Build history of the part. All positions in model axes, mm. A direction names the side the tool comes from. Round coordinates to 2 decimals unless told otherwise and drop trailing zeros. Order: outer loops, then holes, each group sorted by start corner. A loop starts at its lowest first (then second) coordinate and runs counter-clockwise, first axis right, second up. Notation, with made-up numbers: (65, 75) -> (77, 75) arc R31 ccw to (77, 104) -> close; hole circle Ø4 at (32, 3). An arc over 180 degrees is marked (long way). Answer as a JSON object with one key per item and string values.
Autodesk Fusion 360 part; units mm, degrees
sketch "スケッチ1" plane through (0, 0, 0) normal (0, 0, 1) x (1, 0, 0)
  circle A0 centre (0, 0) radius 10
  line L0 (0, 10) -> (12, 10)
  line L1 (12, 10) -> (12, 22)
  line L2 (19, 22) -> (19, -16)
  line L3 (12, -20) -> (12, -10)
  line L4 (12, -10) -> (0, -10)
  line L5 (0, -7) -> (0, 7)
  line L6 (19, -7) -> (14, -7)
  line L7 (14, -7) -> (14, 7)
  line L8 (14, 7) -> (19, 7)
  line L9 (12, 22) -> (19, 22)
  line L10 (12, -20) -> (27, -20)
  line L11 (27, -20) -> (27, -13)
  line L12 (27, -13) -> (23, -13)
  line L13 (23, -13) -> (23, -16)
  line L14 (23, -16) -> (19, -16)
  point P0 (14, 0)
  dimension "d1" = 20
  dimension "d2" = 12
  dimension "d6" = 7
  dimension "d19" = 14
  dimension "d31" = 5
  dimension "d32" = 14
  dimension "d39" = 22
  dimension "d40" = 13
  dimension "d41" = 3
  dimension "d42" = 4
  dimension "d43" = 4
  dimension "d44" = 4
extrude "押し出し1" add sketch "スケッチ1" along normal blind 8 contours A0 | A0 L0 L1 L2 L3 L4 L6 L7 L8 L9 L10 L11 L12 L13 L14
sketch "スケッチ2" plane through (0, 0, 8) normal (0, 0, 1) x (-1, 0, 0)
  circle A0 centre (0, 0) radius 10
  line L0 (-12, 20) -> (-27, 20)
  line L1 (-27, 20) -> (-27, 13)
  line L2 (-27, 13) -> (-23, 13)
  line L3 (-23, 13) -> (-23, 16)
  line L4 (-23, 16) -> (-19, 16)
  line L5 (-19, 16) -> (-19, 7)
  line L6 (-19, -22) -> (-12, -22)
  line L7 (-12, -22) -> (-12, -10)
  line L8 (-12, -10) -> (0, -10)
  arc A1 (0, -10) -> (0, 10) centre (0, 0) ccw
  line L9 (0, 10) -> (-12, 10)
  line L10 (-12, 10) -> (-12, 20)
  line L11 (-19, 7) -> (-14, 7)
  line L12 (-14, 7) -> (-14, -7)
  line L13 (-14, -7) -> (-19, -7)
  line L14 (-19, -7) -> (-19, -22)
extrude "押し出し2" add sketch "スケッチ2" along normal blind 2.5 contours A0 A1
hole "穴1" at (0, 7, 0) at (0, -7, 0) direction (0, 0, 1) diameter 3.2 end through all
hole "穴3" at (0, 0, 0) direction (0, 0, 1) diameter 8 end through all
sketch "スケッチ3" plane through (0, -10, 0) normal (0, -1, 0) x (1, 0, 0)
  line L0 (0, 0) -> (12, 0)
  line L1 (12, 0) -> (12, 8)
  line L2 (12, 8) -> (0, 8)
  line L3 (0, 8) -> (0, 0)
  line L4 (10, 0) -> (4, 4)
  line L5 (4, 4) -> (-15, 4)
  line L6 (-15, 4) -> (-15, 0)
  line L7 (-15, 0) -> (10, 0)
  dimension "d20" = 10
  dimension "d21" = 15
  dimension "d22" = 6
  dimension "d23" = 4
extrude "押し出し3" cut sketch "スケッチ3" against normal through all contours L0 L3 L4 L5 L7 | L3 L5 L6 L7
sketch "スケッチ4" plane through (19, 0, 0) normal (1, 0, 0) x (0, 1, 0)
  line L0 (7, 0) -> (22, 0)
  line L1 (22, 8) -> (7, 8)
  line L2 (22, 4) -> (18, 4)
  line L3 (22, 0) -> (22, 8)
  line L4 (-16, 8) -> (-16, 0)
  line L5 (7, 8) -> (7, 0)
  line L6 (-16, 0) -> (-7, 0)
  line L7 (-7, 0) -> (-7, 8)
  line L8 (-7, 8) -> (-16, 8)
  dimension "d45" = 4
hole "穴2" at (19, 18, 4) direction (-1, 0, 0) diameter 3 depth 11 tip angle 118
thread "ねじ1"
fillet "フィレット1" radius 4 4 edges at (12, 10, 4) (12, -10, 4) (14, -7, 4) (14, 7, 4)
chamfer "面取り2" distance 1 angle 45 1 edges at (23, -13, 4)
1) Cut at D-D, the plane y = 4.5. Give the cut face in (x, z).
Checked values:
{"outline": "(-8.93, 4) -> (4, 4) -> (10, 0) -> (14.29, 0) -> (14.29, 8) -> (8.93, 8) -> (8.93, 10.5) -> (-8.93, 10.5) -> close"}
2) Which spindle directions (+Z, -Z, +X, -X, +Y, -Y) get a long thin tool onto all of the face, cutting with end or side? Do faces 1 (the face through (12, 20, 4)), 2 (the face through (15.203, 5.859, 4.056)), 3 (the face through (19, -11, 4)), 4 (the face through (-4.5, -0.1, 4)), 5 (the face through (5, -10, 5)). Say none if no direction does.
Checked values:
{"face 1": "+Z, -Z, -X, +Y", "face 2": "+Z, -Z, +X", "face 3": "+Z, -Z, +Y", "face 4": "-Z, -X, +Y, -Y", "face 5": "+Z, -Z, -X, -Y"}
3) Flat gauge pins, fed straight in: pin 1 Ø2 at (x, z) = (-0.5, 9.5) entering from +Y; pin 2 Ø1.5 at (x, y) = (14, -1.5) entering from +Z; pin 3 Ø1.8 at (y, z) = (-17.5, 5) entering from -X. Where does each tip first touch, or does it go through?
Checked values:
{"pin 1": "stops at y = 10", "pin 2": "stops at z = 8", "pin 3": "stops at x = 12"}
4) Probe L1, parallel to Y at x = 0, z = 8.5; L2, parallel to X at y = 0, z = 6; L3, parallel to Z at x = 18.5, y = 12. List the from-to ranges inside material, lowest first. Write a range as from..to.
Checked values:
{"L1": "y = -10..-8.6, -5.4..-4, 4..5.4, 8.6..10", "L2": "x = -10..-4, 4..14", "L3": "z = 0..8"}
5) Cut at C-C, the plane x = 13.5. Give the cut face in (y, z).
Checked values:
{"outline": "(-20, 0) -> (22, 0) -> (22, 8) -> (-20, 8) -> close; hole circle Ø3 at (18, 4)"}
6) Cut at B-B, the plane z = 3.5. Give the cut face in (x, y), plus the area to 3 significant figures.
Checked values:
{"outline": "(4.75, -10) -> (8, -10) arc R4 cw to (12, -14) -> (12, -20) -> (27, -20) -> (27, -13) -> (24, -13) -> (23, -14) -> (23, -16) -> (19, -16) -> (19, -7) -> (18, -7) arc R4 cw to (14, -3) -> (14, 3) arc R4 cw to (18, 7) -> (19, 7) -> (19, 16.59) -> (12, 16.59) -> (12, 14) arc R4 cw to (8, 10) -> (4.75, 10) -> close; (12, 19.41) -> (19, 19.41) -> (19, 22) -> (12, 22) -> close", "area": "406 mm²"}
7) Cut at A-A, the plane y = 18. Give the cut face in (x, z).
Checked values:
{"outline": "(12, 0) -> (19, 0) -> (19, 2.5) -> (12, 2.5) -> close; (12, 5.5) -> (19, 5.5) -> (19, 8) -> (12, 8) -> close"}
8) Pull direction Y, two halves, no side cores. Call faces 6 (the face through (19, 15, 4)), 7 (the face through (-0.07, -8.6, 7.3)), 8 (the face through (4, 10, 5)), 9 (the face through (15.141, -5.797, 4.056)): pulls with the +Y half, pulls with the -Y half, needs draft (parallel to the pull), parting line crosses it, or undercut.
Checked values:
{"face 6": "needs draft", "face 7": "undercut", "face 8": "pulls with the +Y half", "face 9": "undercut"}
